```python
from build123d import *

# Parameters (mm, degrees)
PAD_DEPTH    = 3
SKETCH001_W  = 2
SKETCH001_H  = 4.5
PAD001_DEPTH = 4.5
SKETCH002_R  = 1.15
POCKET_DEPTH = 5


with BuildPart() as pocket:
    # Sketch → Pad (new body)
    with BuildSketch(Plane.XY):
        with BuildLine():
            ThreePointArc((-6.324555, 3), (-5.91608, -3.741657), (0, -7))
            Line((0, -7), (0, -9))
            ThreePointArc((0, -9), (-1.25499, -9.678416), (-1.374773, -11.1))
            Line((-2.625227, -11.1), (-1.374773, -11.1))
            ThreePointArc((-2.625227, -11.1), (-4, -9), (-5.374773, -11.1))
            Line((-6.939388, -11.1), (-5.374773, -11.1))
            ThreePointArc((-6.748835, -9.298374), (-6.98336, -10.184459), (-6.939388, -11.1))
            Line((-10.748835, -9.298374), (-6.748835, -9.298374))
            Line((-10.748835, -7.298374), (-10.748835, -9.298374))
            Line((-10.748835, -7.298374), (-9.748835, -7.298374))
            Line((-9.748835, -7.298374), (-9.748835, -8.298374))
            Line((-9.748835, -8.298374), (-8.048835, -8.298374))
            Line((-8.048835, 1.941626), (-8.048835, -8.298374))
            Line((-8.048835, 1.941626), (-9.748835, 1.941626))
            Line((-9.748835, 1.941626), (-9.748835, 0.941626))
            Line((-9.748835, 0.941626), (-10.748835, 0.941626))
            Line((-10.748835, 3), (-10.748835, 0.941626))
            Line((-10.748835, 3), (-6.324555, 3))
        make_face()
    extrude(amount=PAD_DEPTH)

    # Sketch001 → Pad001 (new body)
    with BuildSketch(Plane.XY.offset(3)):
        with Locations((-7.048835, -6.048374)):
            Rectangle(SKETCH001_W, SKETCH001_H)
    extrude(amount=PAD001_DEPTH)

    # Sketch002 → Pocket (cut)
    with BuildSketch(Plane(origin=(-8.048835, 0, 0), x_dir=(0, -1, 0), z_dir=(-1, 0, 0))):
        with Locations((6.048374, 5.25)):
            Circle(SKETCH002_R)
    extrude(amount=-POCKET_DEPTH, mode=Mode.SUBTRACT)


with BuildPart() as fusion:
    # Part__Mirroring: instance of Pocket
    add(pocket.part.mirror(Plane(origin=(0, 0, 0), x_dir=(0, -1, 0), z_dir=(1, 0, 0))))

    # Fusion: union Pocket
    add(pocket.part)


solid = fusion.part
```
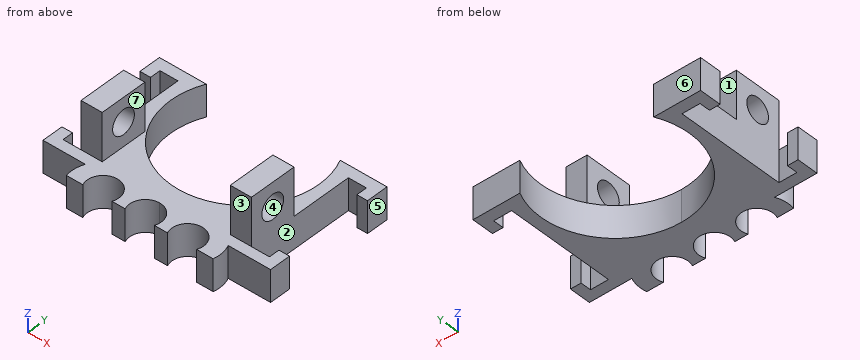
Can you work these out from the model? Positions are in its coordinate system, mm. Face numbers are marked on the shaded views. A direction names the side the tool comes from. Give positions to 0.01 mm unless a question says otherwise; leave off trailing zeros. Write each loop counter-clockwise with the first axis right and the second up, starting at its lowest first coordinate (ties: lowest second). Pieces come first, ordered by that corner, then holes. Notation, with made-up numbers: (36, -15.75) -> (51, -15.75) arc R9 ccw to (51, -5.75) -> close; hole circle Ø2 at (89, 20). An arc over 180 degrees is marked (long way). Write item = value, one per line.
(1) Suppose I cut it at B-B on x = 8.5. Write out the boundary of the cut face in (y, z), then the cut area to 3 significant figures.
Worked out:
outline = (-9.3, 0) -> (-8.3, 0) -> (-8.3, 3) -> (-9.3, 3) -> close; (1.94, 0) -> (3, 0) -> (3, 3) -> (1.94, 3) -> close
area = 6.18 mm^2
(2) Thinking about a two-plate mould opening in X: for the marked faces 5, 6 and 7, which applies, released by +X, released by -X, zero draft, split by the parting line, or undercut?
Worked out:
face_5 = released by +X
face_6 = zero draft
face_7 = undercut
(3) For the marked faces 1, 2, 3 and 4, which set-ups out of +Z, -Z, +X, -X, +Y, -Y let a thin tool reach every point of the face, with its end or its side?
Worked out:
face_1 = +Z, +X, -X, +Y
face_2 = +Z, -Z
face_3 = +Z, +X, -X, -Y
face_4 = +X, -X
(4) I'm going to push flat-ended pins straight in: P1, Ø1, axis at x = 6.5, z = 4.5, coming from the -Y side; P2, Ø3, axis at y = -6.05, z = 5.25, coming from the -X side; P3, Ø2, axis at x = 1, z = 2.5, coming from the +Y side; P4, Ø3, axis at x = 4, z = 6.5, coming from the +Y side. Where does each tip first touch, or does it pass through?
Worked out:
P1 = -8.3
P2 = -8.05
P3 = -6.71
P4 = through
(5) I need wall thicknesses on probe 1 along X at (y, z) = (-10.5, 0.75); probe 2 along X at (y, z) = (-7.75, 1.5); probe 3 along X at (y, z) = (-4.5, 5). Which ranges of each line are inside material? Lowest first, please. Write a range as from..to.
Worked out:
probe_1 = -7..-5.5, -2.5..-1.5, 1.5..2.5, 5.5..7
probe_2 = -10.75..-9.75, -8.05..8.05, 9.75..10.75
probe_3 = -8.05..-6.05, 6.05..8.05
(6) Suppose I cut it at A-A on z = 5.25. Write out the boundary of the cut face in (x, y).
Worked out:
outline = (-8.05, -8.3) -> (-6.05, -8.3) -> (-6.05, -7.2) -> (-8.05, -7.2) -> close; (-8.05, -4.9) -> (-6.05, -4.9) -> (-6.05, -3.8) -> (-8.05, -3.8) -> close; (6.05, -8.3) -> (8.05, -8.3) -> (8.05, -7.2) -> (6.05, -7.2) -> close; (6.05, -4.9) -> (8.05, -4.9) -> (8.05, -3.8) -> (6.05, -3.8) -> close
(7) Suppose I cut it at C-C on z = 3.25. Write out the boundary of the cut face in (x, y).
Worked out:
outline = (-8.05, -8.3) -> (-6.05, -8.3) -> (-6.05, -3.8) -> (-8.05, -3.8) -> close; (6.05, -8.3) -> (8.05, -8.3) -> (8.05, -3.8) -> (6.05, -3.8) -> close
